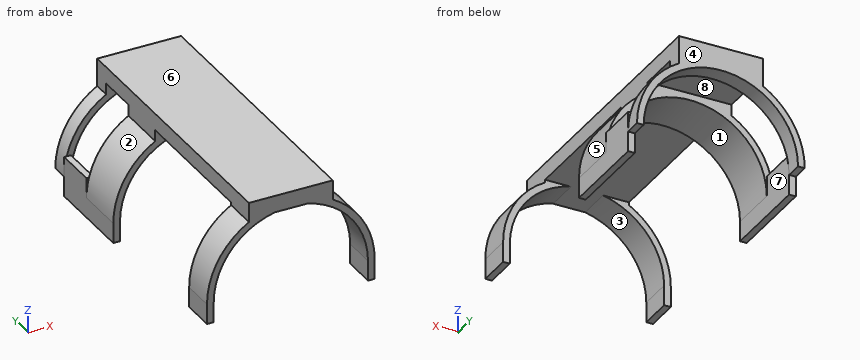
```python
from build123d import *

# Parameters (mm, degrees)
SKETCH_1_W      = 50
SKETCH_1_H      = 10
EXTRUDE_1_DEPTH = 160
EXTRUDE_START   = 105
EXTRUDE_3_DEPTH = 30
EXTRUDE_9_DEPTH = 20
SKETCH_3_W      = 4
SKETCH_3_H      = 24
EXTRUDE_4_DEPTH = 25
EXTRUDE_8_DEPTH = 10


# Read off the part's stored shape, not the designer's step: 凸台-拉伸3
with BuildPart() as part:
    # 草图1 → 凸台-拉伸1 (new body)
    with BuildSketch(Plane(origin=(0, 0, 0), x_dir=(1, 0, 0), z_dir=(0, 1, 0))):
        Rectangle(SKETCH_1_W, SKETCH_1_H)
    extrude(amount=EXTRUDE_1_DEPTH)

    # 凸台-拉伸3 outline → 凸台-拉伸3 (add)
    with BuildSketch(Plane(origin=(0, 0, 0), x_dir=(1, 0, 0), z_dir=(0, 1, 0)).offset(EXTRUDE_START)):
        with BuildLine():
            Line((-25, 11.698729811), (-25, 5))
            Line((-25, 5), (25, 5))
            Line((25, 5), (25, 11.698729811))
            ThreePointArc((25, 11.698729811), (43.301270189, 30), (50, 55))
            Line((50, 55), (50, 67))
            Line((50, 67), (46, 67))
            Line((46, 67), (46, 55))
            ThreePointArc((46, 55), (0, 9), (-46, 55))
            Line((-46, 55), (-46, 67))
            Line((-46, 67), (-50, 67))
            Line((-50, 67), (-50, 55))
            ThreePointArc((-50, 55), (-43.301270189, 30), (-25, 11.698729811))
        make_face()
    extrude(amount=EXTRUDE_3_DEPTH)

    # 草图6 → 凸台-拉伸9 (add)
    with BuildSketch(Plane.XZ):
        with BuildLine():
            Line((-17.162962033, 1.601757508), (17.472067362, 1.754788629))
            Line((17.472067362, 1.754788629), (25, -5))
            Line((25, -5), (25, -6.698729811))
            ThreePointArc((25, -6.698729811), (43.301270189, -25), (50, -50))
            Line((50, -50), (50, -62))
            Line((50, -62), (46, -62))
            Line((46, -62), (46, -50))
            ThreePointArc((46, -50), (0, -4), (-46, -50))
            Line((-46, -50), (-46, -62))
            Line((-46, -62), (-50, -62))
            Line((-50, -62), (-50, -50))
            ThreePointArc((-50, -50), (-43.301270189, -25), (-25, -6.698729811))
            Line((-25, -6.698729811), (-25, -5))
            Line((-25, -5), (-17.162962033, 1.601757508))
        make_face()
    extrude(amount=-EXTRUDE_9_DEPTH)

    # 草图3 → 凸台-拉伸4 (add)
    with BuildSketch(Plane(origin=(0, 135, 0), x_dir=(1, 0, 0), z_dir=(0, 1, 0))):
        with Locations((-48, 55)):
            Rectangle(SKETCH_3_W, SKETCH_3_H)
        with Locations((48, 55)):
            Rectangle(SKETCH_3_W, SKETCH_3_H)
    extrude(amount=EXTRUDE_4_DEPTH)

    # 草图4 → 凸台-拉伸8 (add)
    with BuildSketch(Plane(origin=(0, 160, 0), x_dir=(1, 0, 0), z_dir=(0, 1, 0))):
        with BuildLine():
            Line((-50, 55), (-46, 55))
            ThreePointArc((-46, 55), (0, 9), (46, 55))
            Line((46, 55), (50, 55))
            ThreePointArc((50, 55), (43.301270189, 30), (25, 11.698729811))
            Line((25, 11.698729811), (25, -5))
            Line((25, -5), (-25, -5))
            Line((-25, -5), (-25, 11.698729811))
            ThreePointArc((-25, 11.698729811), (-43.301270189, 30), (-50, 55))
        make_face()
    extrude(amount=EXTRUDE_8_DEPTH)


solid = part.part
```
Work out the finished part from the listing and answer in its coordinate system (mm). Face numbers are marked on the shaded views. A direction names the side the tool comes from. Round coordinates to 2 decimals unless told otherwise and drop trailing zeros. Loops run counter-clockwise (first coordinate to the right, second up) from the corner with the lowest first, then second, coordinate; pieces in that order, holes last.
(1) The part is cut by section D-D, the plane x = 0. Give the vertices of the cut face in (y, z), and give its area (3 significant figures).
Computed values:
outline: (0, -5) - (105, -5) - (105, -9) - (135, -9) - (135, -5) - (160, -5) - (160, -9) - (170, -9) - (170, 5) - (0, 5) - close
area: 1,860 mm2
(2) The part is cut by section A-A, the plane y = 153.5. Give the vertices of the cut face in (x, z).
Computed values:
outline: (-50, -67) - (-46, -67) - (-46, -43) - (-50, -43) - close; (-25, -5) - (25, -5) - (25, 5) - (-25, 5) - close; (46, -67) - (50, -67) - (50, -43) - (46, -43) - close
(3) For the marked faces 5, 6, 7 and 8, determine the directions among +Z, -Z, +X, -X, +Y, -Y from which every point of the face is accessible in a straight line to the end or side of a thin tool.
Computed values:
face 5: +Z, +X
face 6: +Z, +X, -X, +Y, -Y
face 7: -Z
face 8: -Z, +X, -X
(4) The part is cut by section B-B, the plane z = -39. Give the vertices of the cut face in (x, y) (3 decimals).
Computed values:
outline: (-48.775, 0) - (-44.665, 0) - (-44.665, 20) - (-48.775, 20) - close; (-47.371, 105) - (-43.128, 105) - (-43.128, 135) - (-47.371, 135) - close; (-47.371, 160) - (-43.128, 160) - (-43.128, 170) - (-47.371, 170) - close; (43.128, 105) - (47.371, 105) - (47.371, 135) - (43.128, 135) - close; (43.128, 160) - (47.371, 160) - (47.371, 170) - (43.128, 170) - close; (44.665, 0) - (48.775, 0) - (48.775, 20) - (44.665, 20) - close
(5) The part is cut by section C-C, the plane x = -33.5. Give the vertices of the cut face in (y, z), and give its area (3 significant figures).
Computed values:
outline: (0, -18.48) - (20, -18.48) - (20, -12.88) - (0, -12.88) - close; (105, -23.48) - (135, -23.48) - (135, -17.88) - (105, -17.88) - close; (160, -23.48) - (170, -23.48) - (170, -17.88) - (160, -17.88) - close
area: 336 mm2
(6) Find the intervals of material crossed by L1, parallel to X at y = 13, z = -55.5; L2, parallel to Y at x = 44, z = -38.5; L3, parallel to X at y = 89.5, z = -4.5, in increasing order.
Computed values:
L1: x = -50 to -46, 46 to 50
L2: y = 105 to 135, 160 to 170
L3: x = -25 to 25
(7) Each of these flat-tipped pins is pushed along its axis until it touches: P1, Ø2, axis at x = 47.5, y = 151.5, coming from the +Z side; P2, Ø1.2, axis at x = 47.5, y = 162.5, coming from the -Z side; P3, Ø18.5, axis at y = 78, z = -1.5, coming from the +X side; P4, Ø10, axis at x = -27.5, z = -23.5, coming from the +Y side. Where does it stop, or does it pass through?
Computed values:
P1: stops at z = -43
P2: stops at z = -55
P3: stops at x = 25
P4: stops at y = 170
(8) The mould has two halves that part along X. Classify the marked faces 1, 2, 3 and 4: pulls with the +X half, pulls with the -X half, needs draft (parallel to the pull), parting line crosses it, or undercut.
Computed values:
face 1: undercut
face 2: pulls with the -X half
face 3: undercut
face 4: needs draft
